Check sheet for the modelled part. Datum: model origin and axes. Units: mm. A direction names the side the tool comes from. Coordinates: 2 decimals unless noted, no trailing zeros. Write each loop counter-clockwise with the first axis right and the second up, starting at its lowest first coordinate (ties: lowest second). Pieces come first, ordered by that corner, then holes. Notation, with made-up numbers: (-36, -34.5) -> (-5, -34.5) arc R16 cw to (-5, -20.5) -> close; hole circle Ø8 at (-12.75, -15). An arc over 180 degrees is marked (long way). Put each result on its own line as item: value.
```python
from build123d import *

# Parameters (mm, degrees)
EXTRUDE_1_DEPTH     = 15
SKETCH_3_W          = 16
SKETCH_3_H          = 15
EXTRUDE_2_DEPTH     = 4
SKETCH_2_R          = 13.51
CUT_EXTRUDE_2_DEPTH = 13
SKETCH_4_W          = 4.565228969
SKETCH_4_H          = 15
EXTRUDE_3_DEPTH     = 40
FILLET_2_R          = 2
SKETCH_5_R          = 2
EXTRUDE_4_DEPTH     = 2
FILLET_3_R          = 2


with BuildPart() as part:
    # 草图1 → 凸台-拉伸1 (new body)
    with BuildSketch(Plane(origin=(0, 0, 0), x_dir=(1, 0, 0), z_dir=(0, 1, 0))):
        with BuildLine():
            Line((6.148844254, 16.917201729), (-6.148844254, 16.917201729))
            ThreePointArc((-6.148844254, 16.917201729), (0, -18), (6.148844254, 16.917201729))
        make_face()
    extrude(amount=EXTRUDE_1_DEPTH)

    # 草图3 → 凸台-拉伸2 (add)
    with BuildSketch(Plane(origin=(0, 0, -16.917201729), x_dir=(-1, 0, 0), z_dir=(0, 0, -1))):
        with Locations((0, 7.5)):
            Rectangle(SKETCH_3_W, SKETCH_3_H)
    extrude(amount=-EXTRUDE_2_DEPTH)

    # 草图2 → 切除-拉伸2 (cut)
    with BuildSketch(Plane(origin=(0, 15, 0), x_dir=(1, 0, 0), z_dir=(0, 1, 0))):
        with Locations(Location((-0.775740082, 0, 0), (0, 0, 270))):
            Circle(SKETCH_2_R)
    extrude(amount=-CUT_EXTRUDE_2_DEPTH, mode=Mode.SUBTRACT)

    # 草图4 → 凸台-拉伸3 (add)
    with BuildSketch(Plane(origin=(0, 0, -16.917201729), x_dir=(-1, 0, 0), z_dir=(0, 0, -1))):
        with Locations((5.717385516, 7.5)):
            Rectangle(SKETCH_4_W, SKETCH_4_H)
        with Locations((-5.717385516, 7.5)):
            Rectangle(SKETCH_4_W, SKETCH_4_H)
    extrude(amount=EXTRUDE_3_DEPTH)

    # 圆角2
    fillet_2_edges = [part.edges().sort_by_distance(p)[0] for p in [
        (-3.434771031, 7.5, -16.917201729),
        (3.434771031, 7.5, -16.917201729),
    ]]
    fillet(fillet_2_edges, radius=FILLET_2_R)

    # 草图5 → 凸台-拉伸4 (add)
    with BuildSketch(Plane(origin=(0, 0, -56.917201729), x_dir=(-1, 0, 0), z_dir=(0, 0, -1))):
        Polygon((-17.5, 0), (-17.5, 15), (12.5, 15), (17.5, 15), (17.5, 0), (8, 0), align=None)
        with Locations((-12, 7.5)):
            Circle(SKETCH_5_R, mode=Mode.SUBTRACT)
        with Locations((12, 7.5)):
            Circle(SKETCH_5_R, mode=Mode.SUBTRACT)
    extrude(amount=EXTRUDE_4_DEPTH)

    # 圆角3
    fillet_3_edges = [part.edges().sort_by_distance(p)[0] for p in [
        (-3.434771031, 7.5, -56.917201729),
        (3.434771031, 7.5, -56.917201729),
    ]]
    fillet(fillet_3_edges, radius=FILLET_3_R)


solid = part.part
```
Q1. Cross-section at A-A (x = 0). Record the cut outline in (y, z), plus the area to 3 significant figures.
Recorded:
outline: (0, -58.92) -> (15, -58.92) -> (15, -56.92) -> (0, -56.92) -> close; (0, -16.92) -> (15, -16.92) -> (15, -13.49) -> (2, -13.49) -> (2, 13.49) -> (15, 13.49) -> (15, 18) -> (0, 18) -> close
area: 203 mm2
Q2. Material ranges on line 1 along X through (y, z) = (5.75, 0); line 2 along Z through (x, y) = (-1, 13); line 3 along Z through (x, y) = (2, 9.25), recorded low to high.
Recorded:
line 1: x = -18 to -14.29, 12.73 to 18
line 2: z = -58.92 to -56.92, -16.92 to -13.51, 13.51 to 17.97
line 3: z = -58.92 to -56.84, -17 to -13.22, 13.22 to 17.89
Q3. Depth check by flat-ended pin: P1, Ø7.5, axis at x = 11.5, y = 11, coming from the +Z side; P2, Ø4.5, axis at x = -12.5, y = 9.5, coming from the +Z side; P3, Ø4, axis at x = 4.5, y = 7.5, coming from the +Z side. Enter the tip coordinate at first touch or a pass-through.
Recorded:
P1: stops at z = 16.25
P2: stops at z = 14.8
P3: stops at z = 17.83
Q4. Cross-section at D-D (y = 11.25). Record the cut outline in (x, z), plus the area to 3 significant figures.
Recorded:
outline: (-17.5, -58.92) -> (17.5, -58.92) -> (17.5, -56.92) -> (8, -56.92) -> (8, -16.12) arc R18 ccw (long way) to (-8, -16.12) -> (-8, -56.92) -> (-17.5, -56.92) -> close; hole circle Ø27.02 at (-0.78, 0); hole (-3.43, -54.92) arc R2 ccw to (-1.43, -56.92) -> (1.43, -56.92) arc R2 ccw to (3.43, -54.92) -> (3.43, -18.92) arc R2 ccw to (1.43, -16.92) -> (-1.43, -16.92) arc R2 ccw to (-3.43, -18.92) -> close
area: 876 mm2
Q5. Cross-section at C-C (z = 0). Record the cut outline in (x, y).
Recorded:
outline: (-18, 0) -> (18, 0) -> (18, 15) -> (12.73, 15) -> (12.73, 2) -> (-14.29, 2) -> (-14.29, 15) -> (-18, 15) -> close
Q6. Tool access check on faces 1 (the flat face through (-8, 7, -36)), 2 (the flat face through (14, 9, -56.917)), 3 (the flat face through (17.5, 7, -58)), 4 (the flat face through (0, 8, -16.917)). Record the directions out of +Z, -Z, +X, -X, +Y, -Y that give a thin tool (end or side, any length) a straight path to the whole face; none if there is none.
Recorded:
face 1: -X, +Y, -Y
face 2: +X, +Y, -Y
face 3: -Z, +X, +Y, -Y
face 4: +Y, -Y
Q7. Cross-section at B-B (x = 12). Record the cut outline in (y, z), plus the area to 3 significant figures.
Recorded:
outline: (0, -58.92) -> (5.5, -58.92) -> (5.5, -56.92) -> (0, -56.92) -> close; (0, -13.42) -> (15, -13.42) -> (15, -4.39) -> (2, -4.39) -> (2, 4.39) -> (15, 4.39) -> (15, 13.42) -> (0, 13.42) -> close; (9.5, -58.92) -> (15, -58.92) -> (15, -56.92) -> (9.5, -56.92) -> close
area: 310 mm2
Q8. Mould release check, pull along Z, two halves, no side actions. Record for faces 5 (the flat face through (0, 0, -11)), 6 (the flat face through (-3.435, 7, -37)), 7 (the flat face through (0, 8, -58.917)): released by +Z, released by -Z, zero draft, split by the parting line, or undercut.
Recorded:
face 5: zero draft
face 6: undercut
face 7: released by -Z
